from build123d import *

# Parameters (mm, degrees)
F0_R      = 19.5
F1_DEPTH  = 17
F2_R      = 9.5
F3_DEPTH  = 14
F4_R      = 18.5
F4_R_2    = 10.5
F5_DEPTH  = 16
F6_R      = 2
F7_DEPTH  = 25
F8_R      = 3.5
F9_DEPTH  = 10
F10_R     = 2
F11_DEPTH = 10
F12_R     = 4
F13_DEPTH = 1
F14_R     = 2.5
F15_DEPTH = 0.75
F16_R     = 0.5
F17_DEPTH = 0.5
F19_R     = 0.75
F18_R     = 10.5
F18_R_2   = 9.5
F20_DEPTH = 0.25


with BuildPart() as f1:
    # F0 (on Front) → F1 (new body)
    with BuildSketch(Plane.XZ):
        Circle(F0_R)
    extrude(amount=F1_DEPTH)

    # F2 (on face) → F3 (cut)
    with BuildSketch(Plane.XZ.offset(17)):
        Circle(F2_R)
    extrude(amount=-F3_DEPTH, mode=Mode.SUBTRACT)

    # F4 (on face) → F5 (cut)
    with BuildSketch(Plane(origin=(0, 0, 0), x_dir=(-1, 0, 0), z_dir=(0, 1, 0))):
        Circle(F4_R)
        Circle(F4_R_2, mode=Mode.SUBTRACT)
    extrude(amount=-F5_DEPTH, mode=Mode.SUBTRACT)

    # F6 (on face) → F7 (cut)
    with BuildSketch(Plane.XZ.offset(3)):
        with Locations((0, 6.1688632704)):
            Circle(F6_R)
        with Locations((-4.3620450507, 4.3620450507)):
            Circle(F6_R)
        with Locations((-6.1688632704, 0)):
            Circle(F6_R)
        with Locations((-4.3620450507, -4.3620450507)):
            Circle(F6_R)
        with Locations((0, -6.1688632704)):
            Circle(F6_R)
        with Locations((4.3620450507, -4.3620450507)):
            Circle(F6_R)
        with Locations((6.1688632704, 0)):
            Circle(F6_R)
        with Locations((4.3620450507, 4.3620450507)):
            Circle(F6_R)
    extrude(amount=-F7_DEPTH, mode=Mode.SUBTRACT)

    # F8 (on face) → F9 (join)
    with BuildSketch(Plane(origin=(0, 0, 0), x_dir=(-1, 0, 0), z_dir=(0, 1, 0))):
        Circle(F8_R)
    extrude(amount=F9_DEPTH)

    # F10 (on face) → F11 (cut)
    with BuildSketch(Plane(origin=(0, 10, 0), x_dir=(-1, 0, 0), z_dir=(0, 1, 0))):
        Circle(F10_R)
    extrude(amount=-F11_DEPTH, mode=Mode.SUBTRACT)

    # F12 (on face) → F13 (join)
    with BuildSketch(Plane.XZ.offset(3)):
        with Locations((0.0866679911, 0.0506265242)):
            Circle(F12_R)
    extrude(amount=F13_DEPTH)

    # F14 (on face) → F15 (join)
    with BuildSketch(Plane.XZ.offset(4)):
        Circle(F14_R)
    extrude(amount=F15_DEPTH)

    # F16 (on face) → F17 (join)
    with BuildSketch(Plane.XZ.offset(4)):
        with Locations((0, 3.2079922967)):
            Circle(F16_R)
        with Locations((-1.8856105614, 2.5953202858)):
            Circle(F16_R)
        with Locations((-3.050981978, 0.9913241375)):
            Circle(F16_R)
        with Locations((-3.050981978, -0.9913241375)):
            Circle(F16_R)
        with Locations((-1.8856105614, -2.5953202858)):
            Circle(F16_R)
        with Locations((0, -3.2079922967)):
            Circle(F16_R)
        with Locations((1.8856105614, -2.5953202858)):
            Circle(F16_R)
        with Locations((3.050981978, -0.9913241375)):
            Circle(F16_R)
        with Locations((3.050981978, 0.9913241375)):
            Circle(F16_R)
        with Locations((1.8856105614, 2.5953202858)):
            Circle(F16_R)
    extrude(amount=F17_DEPTH)

    # F19
    f19_edges = [f1.edges().sort_by_distance(p)[0] for p in [
        (-19.5, -17, 0),
    ]]
    fillet(f19_edges, radius=F19_R)

    # F18 (on face) → F20 (join)
    with BuildSketch(Plane.XZ.offset(17)):
        Circle(F18_R)
        Circle(F18_R_2, mode=Mode.SUBTRACT)
    extrude(amount=F20_DEPTH)


solid = f1.part
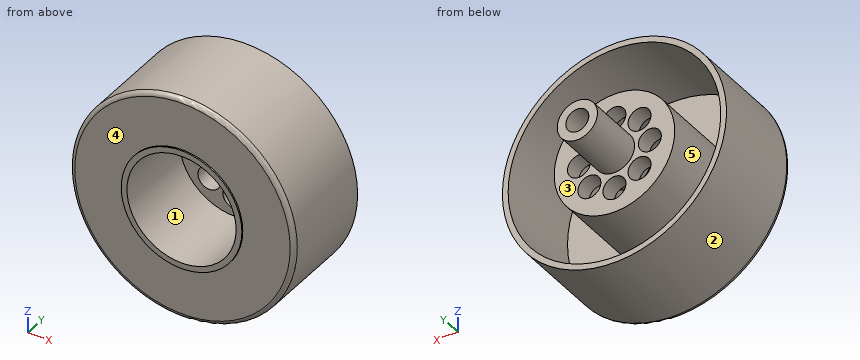
Part model, mm, in its own coordinate system. Face numbers are marked on the shaded views. A direction names the side the tool comes from. Give positions to 0.01 mm unless a question says otherwise; leave off trailing zeros. Loops run counter-clockwise (first coordinate to the right, second up) from the corner with the lowest first, then second, coordinate; pieces in that order, holes last.
(1) Band-saw the part on C-C (y = 8.25). Write the cut outline in (x, z).
Return value:
outline: circle Ø7 at (0, 0); hole circle Ø4 at (0, 0)
(2) 3-axis set-ups, long thin cutter, end or side, ignore diameter. For the marked faces 4 and 5: which of +Z, -Z, +X, -X, +Y, -Y reach the whole face in a straight line?
Return value:
face 4: -Y
face 5: +Y
(3) Band-saw the part on B-B (x = 0). Count the separate pieces of the cut face and the enclosed holes in it, and give its area (3 significant figures).
Return value:
separate pieces: 3
enclosed holes: 0
area: 160 mm2
(4) Drill centre lines: line 1 along Z through (x, y) = (0, -2.4); line 2 along Z through (x, y) = (1, -10.5); line 3 along Z through (x, y) = (-3, -9.75). Where is each one in solid material? Low to high.
Return value:
line 1: z = -19.5 to -18.5, -10.5 to -8.17, -4.17 to 4.17, 8.17 to 10.5, 18.5 to 19.5
line 2: z = -19.47 to -18.47, -10.45 to -9.45, 9.45 to 10.45, 18.47 to 19.47
line 3: z = -19.27 to -18.26, -10.06 to -9.01, 9.01 to 10.06, 18.26 to 19.27
(5) Pin check, flat tips, straight feed: pin 1 (8 mm diameter, centred on y = -14.5, z = 8, fed in from +X); pin 2 (5 mm diameter, centred on x = 4.36, z = 4.36, fed in from -Y); pin 3 (5 mm diameter, centred on x = -6, y = -10.5, fed in from -Z). Stop position of each tip, or through.
Return value:
pin 1: stops at x = 19.09
pin 2: stops at y = -4
pin 3: stops at z = -19.18
(6) Band-saw the part on A-A (y = -14.5). Write the cut outline in (x, z).
Return value:
outline: circle Ø39 at (0, 0); circle Ø21 at (0, 0); hole circle Ø37 at (0, 0); hole circle Ø19 at (0, 0)
(7) Pull direction Z, two halves, no side cores. Call the marked faces 1, 2 and 3: pulls with the +Z half, pulls with the -Z half, needs draft (parallel to the pull), parting line crosses it, or undercut.
Return value:
face 1: undercut
face 2: parting line crosses it
face 3: needs draft
